Read the model definition and answer for the solid it produces. Units are mm, in the model's axes. A direction names the side the tool comes from. Coordinates: 2 decimals unless noted, no trailing zeros. Loops run counter-clockwise (first coordinate to the right, second up) from the corner with the lowest first, then second, coordinate; pieces in that order, holes last.
Q1. Which of the six approach directions +Z, -Z, +X, -X, +Y, -Y give full straight-line access (tool end or side, diameter ignored) to faces 1 (the face through (-5.9, -1.18, -0.03)), 2 (the face through (1, 8.3, 2)), 3 (the face through (8.9, 1.4, 2.7))?
Q2. Flat-ended cylindrical pins translate along their axes: P1, Ø1.1, axis at x = -1.5, z = 3, coming from the +Y side; P2, Ø0.5, axis at x = 4, z = 2.5, coming from the -Y side; P3, Ø0.6, axis at x = 4, z = 2.5, coming from the +Y side. Find the tip coordinate at first contact, or state that the pin passes through.
Q3. Section D-D (x = 0) is taken. Give the vertices of the cut face in (y, z), then the cut area to 3 significant figures.
Q4. Section C-C (z = -1) is taken. Give the vertices of the cut face in (x, y), then the cut area to 3 significant figures.
Q5. Straight lines are drawn through the part: line 1 (Z direction, x = 2, y = 5.5); line 2 (Y direction, x = -5, z = 2.25); line 3 (Y direction, x = 9.5, z = 2). For each, find the intervals that lie inside material, in ascending order.
Q6. Section B-B (x = -9) is taken. Give the vertices of the cut face in (y, z), then the cut area to 3 significant figures.
Q7. The mould has two halves that part along X. Classify faces 4 (the face through (10.293, 4, 0)), 5 (the face through (9, 8.3, 2)): pulls with the +X half, pulls with the -X half, needs draft (parallel to the pull), parting line crosses it, or undercut.
Q8. Section A-A (z = 2.5) is taken. Count the separate pieces of the cut face and the enclosed holes in it, then the cut area to 3 significant figures.
from build123d import *

# Parameters (mm, degrees)
SKETCH2_W           = 20.586666666
SKETCH2_H           = 6.3
BOSS_EXTRUDE1_DEPTH = 8.8
SKETCH3_R           = 0.4
BOSS_EXTRUDE2_DEPTH = 2.4
SKETCH4_W           = 1.405361948
SKETCH4_H           = 6
CUT_EXTRUDE1_DEPTH  = 1
SKETCH5_W           = 1.27
SKETCH5_H           = 1.5
CUT_EXTRUDE2_DEPTH  = 0.5
LPATTERN1_COUNT     = 8
LPATTERN1_PITCH     = 2.54


with BuildPart() as part:
    # Sketch2 → Boss-Extrude1 (new body)
    with BuildSketch(Plane(origin=(0, 0, 0), x_dir=(1, 0, 0), z_dir=(0, 1, 0))):
        Rectangle(SKETCH2_W, SKETCH2_H)
    extrude(amount=BOSS_EXTRUDE1_DEPTH)

    # Sketch3 → Boss-Extrude2 (add)
    with BuildSketch(Plane.XZ):
        with Locations((-8.823333333, -0.15)):
            Circle(SKETCH3_R)
    boss_extrude2 = extrude(amount=BOSS_EXTRUDE2_DEPTH)

    # Sketch4 → Cut-Extrude1 (cut)
    with BuildSketch(Plane.XY.offset(3.15)):
        with Locations((-8.823333333, 4.4)):
            Rectangle(SKETCH4_W, SKETCH4_H)
    cut_extrude1 = extrude(amount=-CUT_EXTRUDE1_DEPTH, mode=Mode.SUBTRACT)

    # Sketch5 → Cut-Extrude2 (cut)
    with BuildSketch(Plane(origin=(0, 8.8, 0), x_dir=(1, 0, 0), z_dir=(0, 1, 0))):
        with Locations((-8.823333333, -2.4)):
            Rectangle(SKETCH5_W, SKETCH5_H)
    cut_extrude2 = extrude(amount=-CUT_EXTRUDE2_DEPTH, mode=Mode.SUBTRACT)

    # LPattern1: Boss-Extrude2, Cut-Extrude1, Cut-Extrude2 ×8
    with Locations(*[(i * LPATTERN1_PITCH, 0, 0) for i in range(1, LPATTERN1_COUNT)]):
        add(boss_extrude2)
        add(cut_extrude1, mode=Mode.SUBTRACT)
        add(cut_extrude2, mode=Mode.SUBTRACT)


solid = part.part
Numbers:
1. face 1: -Y
1. face 2: +Z, +Y
1. face 3: +Z
2. P1: stops at y = 8.8
2. P2: stops at y = 0
2. P3: stops at y = 8.3
3. outline: (0, -3.15) - (8.8, -3.15) - (8.8, 3.15) - (0, 3.15) - close
3. area: 55.4 mm2
4. outline: (-10.29, 0) - (10.29, 0) - (10.29, 8.8) - (-10.29, 8.8) - close
4. area: 181 mm2
5. line 1: z = -3.15 to 2.15
5. line 2: y = 0 to 8.8
5. line 3: y = 0 to 8.3
6. outline: (-2.4, -0.51) - (0, -0.51) - (0, -3.15) - (8.8, -3.15) - (8.8, 1.65) - (8.3, 1.65) - (8.3, 3.15) - (7.4, 3.15) - (7.4, 2.15) - (1.4, 2.15) - (1.4, 3.15) - (0, 3.15) - (0, 0.21) - (-2.4, 0.21) - close
6. area: 50.4 mm2
7. face 4: pulls with the +X half
7. face 5: undercut
8. separate pieces: 1
8. enclosed holes: 8
8. area: 109 mm2
